Input: dimensioned drawing with shaded views. Units: mm. Origin: part minimum x, y, z. Coordinates: 2 decimals unless noted, no trailing zeros. Loops run counter-clockwise (first coordinate to the right, second up) from the corner with the lowest first, then second, coordinate; pieces in that order, holes last. Notation, with made-up numbers: (48, -25) -> (55, -25) arc R21 cw to (55, 9) -> close; hole circle Ø3 at (34.25, 40.25). An arc over 180 degrees is marked (long way). Answer as CSV lines item,"result".
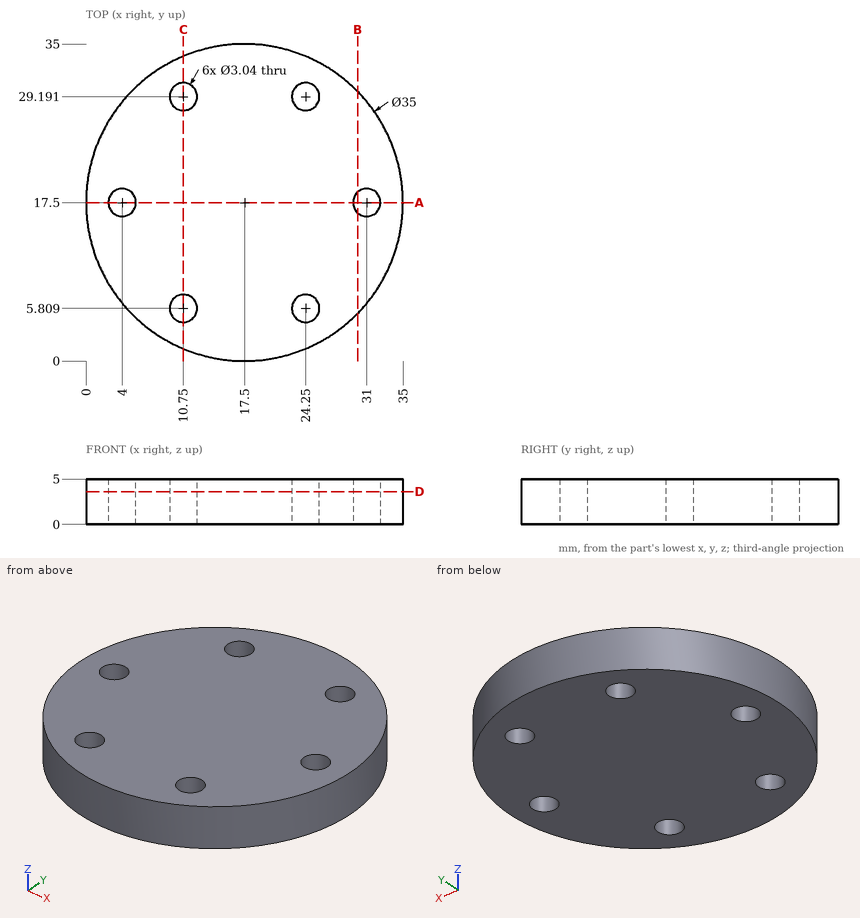
(1) Pin query (flat end, axial travel): pin 1 Ø1 at (x, z) = (27, 3.5) entering from -Y; pin 2 Ø2 at (x, z) = (22, 1.5) entering from +Y; pin 3 Ø2 at (x, z) = (28, 0.5) entering from +Y. Return the tip coordinate at first contact, or that it passes through.
Computed values:
pin 1,"y = 2.49"
pin 2,"y = 34.65"
pin 3,"y = 32.2"
(2) Cut plane B-B (x = 30). Return the cut outline in (y, z) (1 decimal).
Computed values:
outline,"(5.3, 0) -> (16.4, 0) -> (16.4, 5) -> (5.3, 5) -> close; (18.6, 0) -> (29.7, 0) -> (29.7, 5) -> (18.6, 5) -> close"
(3) Cut plane A-A (y = 17.5). Return the cut outline in (x, z), then the cut area to 3 significant figures.
Computed values:
outline,"(0, 0) -> (2.48, 0) -> (2.48, 5) -> (0, 5) -> close; (5.52, 0) -> (29.48, 0) -> (29.48, 5) -> (5.52, 5) -> close; (32.52, 0) -> (35, 0) -> (35, 5) -> (32.52, 5) -> close"
area,"145 mm^2"
(4) Cut plane D-D (z = 3.6). Return the cut outline in (x, y).
Computed values:
outline,"circle Ø35 at (17.5, 17.5); hole circle Ø3.04 at (4, 17.5); hole circle Ø3.04 at (10.75, 5.81); hole circle Ø3.04 at (10.75, 29.19); hole circle Ø3.04 at (24.25, 5.81); hole circle Ø3.04 at (24.25, 29.19); hole circle Ø3.04 at (31, 17.5)"
(5) Material intervals for L1, parallel to Y at x = 24.25, z = 3.8 (1 decimal); L2, parallel to Y at x = 24, z = 4.5; L3, parallel to Y at x = 4, z = 2.8 (1 decimal), sorted ascending. Write a range as [from, to].
Computed values:
L1,"[1.4, 4.3], [7.3, 27.7], [30.7, 33.6]"
L2,"[1.25, 4.31], [7.31, 27.69], [30.69, 33.75]"
L3,"[6.4, 16], [19, 28.6]"
(6) Cut plane C-C (x = 10.75). Return the cut outline in (y, z).
Computed values:
outline,"(1.35, 0) -> (4.29, 0) -> (4.29, 5) -> (1.35, 5) -> close; (7.33, 0) -> (27.67, 0) -> (27.67, 5) -> (7.33, 5) -> close; (30.71, 0) -> (33.65, 0) -> (33.65, 5) -> (30.71, 5) -> close"
